Could you check a few things on this model? Use its own coordinates, in mm. A direction names the side the tool comes from. Round coordinates to 2 decimals unless told otherwise and drop trailing zeros. Order: outer loops, then holes, each group sorted by start corner. A loop starts at its lowest first (then second) coordinate and runs counter-clockwise, first axis right, second up. Notation, with made-up numbers: (-0.5, 73.25) - (3.5, 73.25) arc R7 cw to (3.5, 82.25) - close; hole circle Ø6 at (62, 19.5). An arc over 180 degrees is marked (long way). Return JSON: item names as keys, results as strings. Group by question number.
from build123d import *

# Parameters (mm, degrees)
BOSS_EXTRU_1_DEPTH      = 15
ESQUISSE2_W             = 42
ESQUISSE2_H             = 22
ENL_V_MAT_EXTRU_1_DEPTH = 48.36032094485848
ESQUISSE4_R             = 2.1499999999999972
ESQUISSE4_R_2           = 2.1499999999999977
ESQUISSE4_R_3           = 2.1500000000000012
ENL_V_MAT_EXTRU_2_DEPTH = 3
ESQUISSE5_W             = 4
ESQUISSE5_H             = 6.35
ENL_V_MAT_EXTRU_3_DEPTH = 6
ENL_V_MAT_EXTRU_4_DEPTH = 8
BOSS_EXTRU_6_START      = 20
ESQUISSE10_W            = 12.000000000000007
ESQUISSE10_H            = 10.265502917405067
BOSS_EXTRU_6_DEPTH      = 20
ESQUISSE11_W            = 42
ESQUISSE11_H            = 10.265502917405069
BOSS_EXTRU_7_DEPTH      = 5
BOSS_EXTRU_8_DEPTH      = 2.5
BOSS_EXTRU_8_DEPTH_BACK = 35
ESQUISSE13_R            = 1.5500000000000012
ENL_V_MAT_EXTRU_5_DEPTH = 59.51709152034131
BOSS_EXTRU_9_DEPTH      = 2.5
CONG_1_R                = 1
ESQUISSE15_R            = 1.4999999999999987
BOSS_EXTRU_10_DEPTH     = 8
CONG_2_R                = 3.5


with BuildPart() as part:
    # Esquisse1 → Boss.-Extru.1 (new body)
    with BuildSketch(Plane.XY):
        with BuildLine():
            Line((30, -12.999999999999996), (-30, -13.000000000000004))
            Line((-30, -13.000000000000004), (-30, 12.999999999999996))
            Line((-30, 12.999999999999996), (30, 13.000000000000004))
            ThreePointArc((30, 13.000000000000004), (43.00000000000001, 3.47e-15), (30, -12.999999999999996))
        make_face()
    extrude(amount=BOSS_EXTRU_1_DEPTH)

    # Esquisse2 → Enlèv. mat.-Extru.1 (cut, through all)
    with BuildSketch(Plane.XY.offset(15)):
        with Locations((3.0000000000000053, 0)):
            Rectangle(ESQUISSE2_W, ESQUISSE2_H)
    extrude(amount=-ENL_V_MAT_EXTRU_1_DEPTH, mode=Mode.SUBTRACT)

    # Esquisse4 → Enlèv. mat.-Extru.2 (cut)
    with BuildSketch(Plane.XY.offset(15)):
        with Locations((-20.809999999999974, 4.934999999999995)):
            Circle(ESQUISSE4_R)
        with Locations((-20.809999999999974, -4.935000000000005)):
            Circle(ESQUISSE4_R_2)
        with Locations((28.490000000000016, 4.934999999999976)):
            Circle(ESQUISSE4_R_3)
        with Locations((28.490000000000016, -4.93499999999999)):
            Circle(ESQUISSE4_R_3)
    extrude(amount=-ENL_V_MAT_EXTRU_2_DEPTH, mode=Mode.SUBTRACT)

    # Esquisse5 → Enlèv. mat.-Extru.3 (cut)
    with BuildSketch(Plane(origin=(-17.999999999999996, 0, 0), x_dir=(0, 0, -1), z_dir=(1, 0, 0))):
        with Locations((-10, -4.825)):
            Rectangle(ESQUISSE5_W, ESQUISSE5_H)
        with Locations((-10, 4.825)):
            Rectangle(ESQUISSE5_W, ESQUISSE5_H)
    extrude(amount=-ENL_V_MAT_EXTRU_3_DEPTH, mode=Mode.SUBTRACT)

    # Esquisse6 → Enlèv. mat.-Extru.4 (cut)
    with BuildSketch(Plane.ZY.offset(-24.000000000000007)):
        Polygon((12, 8), (8, 8), (8, 1.65), (12, 1.6500000000000004), align=None)
        Polygon((12, -1.6500000000000004), (8, -1.65), (8, -8), (12, -8), align=None)
    extrude(amount=-ENL_V_MAT_EXTRU_4_DEPTH, mode=Mode.SUBTRACT)

    # Esquisse10 → Boss.-Extru.6 (add)
    with BuildSketch(Plane(origin=(0, 0, 0), x_dir=(-1, 0, 0), z_dir=(0, 0, -1)).offset(BOSS_EXTRU_6_START)):
        with Locations((24, 0)):
            Rectangle(ESQUISSE10_W, ESQUISSE10_H)
        with BuildLine():
            Line((-24.000000000000007, 5.1327514587025345), (-41.94382109976481, 5.132751458702534))
            ThreePointArc((-41.94382109976481, 5.132751458702534), (-43, -7.1e-16), (-41.94382109976481, -5.132751458702534))
            Line((-41.94382109976481, -5.132751458702534), (-24.000000000000007, -5.132751458702534))
            Line((-24.000000000000007, -5.132751458702534), (-24.000000000000007, 5.1327514587025345))
        make_face()
    extrude(amount=-BOSS_EXTRU_6_DEPTH)

    # Esquisse11 → Boss.-Extru.7 (add)
    with BuildSketch(Plane(origin=(0, 0, -20), x_dir=(-1, 0, 0), z_dir=(0, 0, -1))):
        with Locations((-3.0000000000000053, 4.4e-16)):
            Rectangle(ESQUISSE11_W, ESQUISSE11_H)
    extrude(amount=-BOSS_EXTRU_7_DEPTH)

    # Esquisse12 → Boss.-Extru.8 (add, two sides: drawn at the far end of the back side and taken through both)
    with BuildSketch(Plane(origin=(0, 0, -20), x_dir=(-1, 0, 0), z_dir=(0, 0, -1)).offset(-BOSS_EXTRU_8_DEPTH_BACK)):
        with BuildLine():
            Line((-29.999999999999993, -12.999999999999996), (-30, 13.000000000000004))
            ThreePointArc((-30, 13.000000000000004), (-37.151021991186546, 10.8564674034221), (-41.94382109976481, 5.132751458702534))
            ThreePointArc((-41.94382109976481, 5.132751458702534), (-43, 5.06e-15), (-41.94382109976481, -5.132751458702532))
            ThreePointArc((-41.94382109976481, -5.132751458702532), (-37.15102199118654, -10.856467403422094), (-29.999999999999993, -12.999999999999996))
        make_face()
    extrude(amount=BOSS_EXTRU_8_DEPTH + BOSS_EXTRU_8_DEPTH_BACK)

    # Esquisse13 → Enlèv. mat.-Extru.5 (cut, through all)
    with BuildSketch(Plane.XY.offset(15)):
        with Locations((36.030874159306855, 4.6664949567902845)):
            Circle(ESQUISSE13_R)
        with Locations((36.030874159306855, -5.3335050432097155)):
            Circle(ESQUISSE13_R)
    extrude(amount=-ENL_V_MAT_EXTRU_5_DEPTH, mode=Mode.SUBTRACT)

    # Esquisse14 → Boss.-Extru.9 (add)
    with BuildSketch(Plane.XY.offset(15)):
        with BuildLine():
            Line((33.160130873307615, 12.610058400482057), (33.160130873307615, -12.610058400482053))
            ThreePointArc((33.160130873307615, -12.610058400482053), (43.00000000000001, 3.47e-15), (33.160130873307615, 12.610058400482057))
        make_face()
    extrude(amount=BOSS_EXTRU_9_DEPTH)

    # Congé1
    cong_1_edges = [part.edges().sort_by_distance(p)[0] for p in [
        (33.160130873307615, 1.78e-15, 15),
    ]]
    fillet(cong_1_edges, radius=CONG_1_R)

    # Esquisse15 → Boss.-Extru.10 (add)
    with BuildSketch(Plane(origin=(0, 0, -20), x_dir=(-1, 0, 0), z_dir=(0, 0, -1))):
        with Locations((6.410000000000011, 6.006e-14)):
            Circle(ESQUISSE15_R)
    extrude(amount=BOSS_EXTRU_10_DEPTH)

    # Congé2
    cong_2_edges = [part.edges().sort_by_distance(p)[0] for p in [
        (-4.910000000000013, 6.024e-14, -20),
    ]]
    fillet(cong_2_edges, radius=CONG_2_R)


solid = part.part
1) I want a section at B-B, the plane z = -21.5. List the corners of the cut face in (x, y) for me.
2) I want a section at D-D, the plane z = 6. List the corners of the cut face in (x, y) for me.
3) I want a section at A-A, the plane x = 23. List the corners of the cut face in (y, z) for me.
4) If I drill on line 1 along Y through (x, z) = (-15.5, 5); line 2 along X through (y, z) = (-6.75, 3.5); line 3 along Y through (x, z) = (-20, 13), over which ranges is the centre line in solid material (lowest first)? Write a range as from..to.
5) We'd pull the mould along X, two halves only. Please class faces 6 (the flat face through (-6, 12, 0)), 7 (the cylindrical face through (-4.91, 0.07, -25.72)), 8 (the flat face through (30, 5, 11)): +X half, -X half, draft (parallel to the pull), parting line (faces both ways), or undercut.
6) Will these pins go through, and if not, where does the flat tip stop? pin 1 (10 mm diameter, centred on x = -4, y = -2, fed in from +Z); pin 2 (8 mm diameter, centred on x = 9.5, z = -13.5, fed in from -Y); pin 3 (4 mm diameter, centred on x = -20.81, y = 4.935, fed in from -Z).
7) For faces 1 (the flat face through (36, 5, 15)), 2 (the flat face through (0, -13, 7)), 3 (the flat face through (0, 13, 7)), 4 (the cylindrical face through (26.34, -4.86, 13.52)), 5 (the flat face through (-21, 8, 10)), which set-ups out of +Z, -Z, +X, -X, +Y, -Y let a thin tool reach every point of the face, with its end or its side?
8) I want a section at C-C, the plane z = 11. List the corners of the cut face in (x, y) for me, plus the area to 3 significant figures.
Outcome:
{
 "1": {"outline": "circle Ø4.26 at (-6.41, 0); (30, -13) arc R13 ccw to (30, 13) - close; hole circle Ø3.1 at (36.03, -5.33); hole circle Ø3.1 at (36.03, 4.67)"},
 "2": {"outline": "(-30, -13) - (30, -13) arc R13 ccw to (30, 13) - (-30, 13) - close; hole (-18, -11) - (24, -11) - (24, 11) - (-18, 11) - close; hole circle Ø3.1 at (36.03, -5.33); hole circle Ø3.1 at (36.03, 4.67)"},
 "3": {"outline": "(-13, 0) - (-11, 0) - (-11, 15) - (-13, 15) - close; (-5.13, -20) - (5.13, -20) - (5.13, -15) - (-5.13, -15) - close; (11, 0) - (13, 0) - (13, 15) - (11, 15) - close"},
 "4": {"line 1": "-13..-11, 11..13", "line 2": "-30..-18, 24..35.4, 36.66..41.11", "line 3": "-13..-6.93, -2.94..2.94, 6.93..13"},
 "5": {"face 6": "draft", "face 7": "parting line", "face 8": "undercut"},
 "6": {"pin 1": "z = -15", "pin 2": "y = -5.13", "pin 3": "z = -20"},
 "7": {"face 1": "-Z", "face 2": "+Z, -Z, +X, -X, -Y", "face 3": "+Z, -Z, +X, -X, +Y", "face 4": "+Z", "face 5": "none"},
 "8": {"outline": "(-30, -13) - (30, -13) arc R13 ccw to (30, 13) - (-30, 13) - close; hole (-24, -8) - (-18, -8) - (-18, -11) - (24, -11) - (24, -8) - (30, -8) - (30, -1.65) - (24, -1.65) - (24, 1.65) - (30, 1.65) - (30, 8) - (24, 8) - (24, 11) - (-18, 11) - (-18, 8) - (-24, 8) - (-24, 1.65) - (-18, 1.65) - (-18, -1.65) - (-24, -1.65) - close; hole circle Ø3.1 at (36.03, -5.33); hole circle Ø3.1 at (36.03, 4.67)", "area": "734 mm^2"}
}
